Part model, mm, in its own coordinate system. Give positions to 0.01 mm unless a question says otherwise; leave off trailing zeros. Order: outer loops, then holes, each group sorted by start corner. A loop starts at its lowest first (then second) coordinate and runs counter-clockwise, first axis right, second up. Notation, with made-up numbers: M 65.5,13.5 L 78.5,13.5 A27 cw 78.5,35.5 Z; hole C 64,27.25 d5. An arc over 180 degrees is marked long. Answer as a JSON object with one key per item and string values.
from build123d import *

# Parameters (mm, degrees)
SKETCH2_R           = 1.65
SKETCH2_R_2         = 11
SKETCH2_R_3         = 2.25
BOSS_EXTRUDE1_DEPTH = 3.8


with BuildPart() as part:
    # Sketch2 → Boss-Extrude1 (new body)
    with BuildSketch(Plane.XY):
        with BuildLine():
            Line((-160, 155), (-87, 155))
            ThreePointArc((-87, 155), (-85.585786438, 154.414213562), (-85, 153))
            Line((-85, 153), (-85, 74.308795954))
            ThreePointArc((-85, 74.308795954), (-84.414213562, 72.894582392), (-83, 72.308795954))
            Line((-83, 72.308795954), (83, 72.308795954))
            ThreePointArc((83, 72.308795954), (84.414213562, 72.894582392), (85, 74.308795954))
            Line((85, 74.308795954), (85, 153))
            ThreePointArc((85, 153), (85.585786438, 154.414213562), (87, 155))
            Line((87, 155), (160, 155))
            Line((160, 155), (160, 55))
            Line((160, 55), (155, 55))
            Line((155, 55), (155, -5))
            Line((155, -5), (160, -5))
            Line((160, -5), (160, -105))
            Line((160, -105), (87, -105))
            ThreePointArc((87, -105), (85.585786438, -104.414213562), (85, -103))
            Line((85, -103), (85, -22))
            ThreePointArc((85, -22), (84.414213562, -20.585786438), (83, -20))
            Line((83, -20), (-83, -20))
            ThreePointArc((-83, -20), (-84.414213562, -20.585786438), (-85, -22))
            Line((-85, -22), (-85, -103))
            ThreePointArc((-85, -103), (-85.585786438, -104.414213562), (-87, -105))
            Line((-87, -105), (-160, -105))
            Line((-160, -105), (-160, -5))
            Line((-160, -5), (-155, -5))
            Line((-155, -5), (-155, 55))
            Line((-155, 55), (-160, 55))
            Line((-160, 55), (-160, 155))
        make_face()
        with Locations(Location((-108.992804496, 124.770936608, 0), (0, 0, 180))):
            Circle(SKETCH2_R, mode=Mode.SUBTRACT)
        with Locations(Location((-108.992804496, 96.101330956, 0), (0, 0, 180))):
            Circle(SKETCH2_R, mode=Mode.SUBTRACT)
        with Locations(Location((108.992804496, 124.770936608, 0), (0, 0, 180))):
            Circle(SKETCH2_R, mode=Mode.SUBTRACT)
        with Locations(Location((108.992804496, 96.101330956, 0), (0, 0, 180))):
            Circle(SKETCH2_R, mode=Mode.SUBTRACT)
        with Locations(Location((108.992804496, 110.436133782, 0), (0, 0, 180))):
            Circle(SKETCH2_R_2, mode=Mode.SUBTRACT)
        with Locations(Location((-108.992804496, 110.436133782, 0), (0, 0, 180))):
            Circle(SKETCH2_R_2, mode=Mode.SUBTRACT)
        with Locations(Location((143.59774802, -0.5, 0), (0, 0, 180))):
            Circle(SKETCH2_R, mode=Mode.SUBTRACT)
        with Locations(Location((143.59774802, 50.5, 0), (0, 0, 180))):
            Circle(SKETCH2_R, mode=Mode.SUBTRACT)
        with Locations(Location((-143.59774802, -0.5, 0), (0, 0, 180))):
            Circle(SKETCH2_R, mode=Mode.SUBTRACT)
        with Locations(Location((-143.59774802, 50.5, 0), (0, 0, 180))):
            Circle(SKETCH2_R, mode=Mode.SUBTRACT)
        with Locations(Location((-47, 10.055, 0), (0, 0, 180))):
            Circle(SKETCH2_R_3, mode=Mode.SUBTRACT)
        with Locations(Location((-47, 39.945, 0), (0, 0, 180))):
            Circle(SKETCH2_R_3, mode=Mode.SUBTRACT)
        with Locations(Location((-71.06, 39.945, 0), (0, 0, 180))):
            Circle(SKETCH2_R_3, mode=Mode.SUBTRACT)
        with Locations(Location((-71.06, 10.055, 0), (0, 0, 180))):
            Circle(SKETCH2_R_3, mode=Mode.SUBTRACT)
        with Locations(Location((71.06, 10.055, 0), (0, 0, 180))):
            Circle(SKETCH2_R_3, mode=Mode.SUBTRACT)
        with Locations(Location((47, 10.055, 0), (0, 0, 180))):
            Circle(SKETCH2_R_3, mode=Mode.SUBTRACT)
        with Locations(Location((47, 39.945, 0), (0, 0, 180))):
            Circle(SKETCH2_R_3, mode=Mode.SUBTRACT)
        with Locations(Location((71.06, 39.945, 0), (0, 0, 180))):
            Circle(SKETCH2_R_3, mode=Mode.SUBTRACT)
        with Locations(Location((108.992804496, -74.770936608, 0), (0, 0, 180))):
            Circle(SKETCH2_R, mode=Mode.SUBTRACT)
        with Locations(Location((108.992804496, -46.101330956, 0), (0, 0, 180))):
            Circle(SKETCH2_R, mode=Mode.SUBTRACT)
        with Locations(Location((108.992804496, -60.436133782, 0), (0, 0, 180))):
            Circle(SKETCH2_R_2, mode=Mode.SUBTRACT)
        with Locations(Location((-108.992804496, -60.436133782, 0), (0, 0, 180))):
            Circle(SKETCH2_R_2, mode=Mode.SUBTRACT)
        with Locations(Location((-108.992804496, -46.101330956, 0), (0, 0, 180))):
            Circle(SKETCH2_R, mode=Mode.SUBTRACT)
        with Locations(Location((-108.992804496, -74.770936608, 0), (0, 0, 180))):
            Circle(SKETCH2_R, mode=Mode.SUBTRACT)
        with Locations(Location((38.179918963, -11.563765186, 0), (0, 0, 180))):
            Circle(SKETCH2_R_3, mode=Mode.SUBTRACT)
        with Locations(Location((-38.179918963, -11.563765186, 0), (0, 0, 180))):
            Circle(SKETCH2_R_3, mode=Mode.SUBTRACT)
        with BuildLine():
            Line((-84, 62.171403079), (-129.59774802, 62.171403079))
            ThreePointArc((-129.59774802, 62.171403079), (-132.426175145, 60.999830204), (-133.59774802, 58.171403079))
            Line((-133.59774802, 58.171403079), (-133.59774802, -8.171403079))
            ThreePointArc((-133.59774802, -8.171403079), (-132.426175145, -10.999830204), (-129.59774802, -12.171403079))
            Line((-129.59774802, -12.171403079), (-84, -12.171403079))
            ThreePointArc((-84, -12.171403079), (-81.171572875, -10.999830204), (-80, -8.171403079))
            Line((-80, -8.171403079), (-80, 58.171403079))
            ThreePointArc((-80, 58.171403079), (-81.171572875, 60.999830204), (-84, 62.171403079))
        make_face(mode=Mode.SUBTRACT)
        with BuildLine():
            Line((84, 62.171403079), (129.59774802, 62.171403079))
            ThreePointArc((129.59774802, 62.171403079), (132.426175145, 60.999830204), (133.59774802, 58.171403079))
            Line((133.59774802, 58.171403079), (133.59774802, -8.171403079))
            ThreePointArc((133.59774802, -8.171403079), (132.426175145, -10.999830204), (129.59774802, -12.171403079))
            Line((129.59774802, -12.171403079), (84, -12.171403079))
            ThreePointArc((84, -12.171403079), (81.171572875, -10.999830204), (80, -8.171403079))
            Line((80, -8.171403079), (80, 58.171403079))
            ThreePointArc((80, 58.171403079), (81.171572875, 60.999830204), (84, 62.171403079))
        make_face(mode=Mode.SUBTRACT)
    extrude(amount=BOSS_EXTRUDE1_DEPTH)


solid = part.part
1. Cut at C-C on y = 19.5. Give the cut face in (x, z).
Worked answers:
{"outline": "M -155,0 L -133.6,0 L -133.6,3.8 L -155,3.8 Z; M -80,0 L 80,0 L 80,3.8 L -80,3.8 Z; M 133.6,0 L 155,0 L 155,3.8 L 133.6,3.8 Z"}
2. Pin check, flat tips, straight feed: P1, Ø1, axis at x = -26, z = 1, coming from the -Y side; P2, Ø3.5, axis at x = 47, y = 10.055, coming from the -Z side; P3, Ø1.5, axis at x = -31.5, z = 2, coming from the +Y side. Stop position of each tip, or through.
Worked answers:
{"P1": "stops at y = -20", "P2": "passes through", "P3": "stops at y = 72.31"}
3. Cut at A-A on x = -93. Give the cut face in (y, z).
Worked answers:
{"outline": "M -105,0 L -12.17,0 L -12.17,3.8 L -105,3.8 Z; M 62.17,0 L 155,0 L 155,3.8 L 62.17,3.8 Z"}
4. Cut at B-B on y = 78. Give the cut face in (x, z), plus the area to 3 significant figures.
Worked answers:
{"outline": "M -160,0 L -85,0 L -85,3.8 L -160,3.8 Z; M 85,0 L 160,0 L 160,3.8 L 85,3.8 Z", "area": "570 mm^2"}
5. Cut at D-D on y = 114.5. Give the cut face in (x, z).
Worked answers:
{"outline": "M -160,0 L -119.21,0 L -119.21,3.8 L -160,3.8 Z; M -98.77,0 L -85,0 L -85,3.8 L -98.77,3.8 Z; M 85,0 L 98.77,0 L 98.77,3.8 L 85,3.8 Z; M 119.21,0 L 160,0 L 160,3.8 L 119.21,3.8 Z"}
6. Two-plate mould, pull along X, no slides. Class faces 1 (the cylindrical face through (117.1, 103, 1.9)), 2 (the flat face through (2, 27, 3.8)): +X half, -X half, draft (parallel to the pull), parting line (faces both ways), or undercut.
Worked answers:
{"face 1": "undercut", "face 2": "draft"}
7. Probe line 1 along X through (y, z) = (23.5, 3.1); line 2 along Y through (x, z) = (-46.5, 3.55); line 3 along X through (y, z) = (109.5, 2.15). List the from-to ranges inside material, lowest first.
Worked answers:
{"line 1": "x = -155 to -133.6, -80 to 80, 133.6 to 155", "line 2": "y = -20 to 7.86, 12.25 to 37.75, 42.14 to 72.31", "line 3": "x = -160 to -119.95, -98.03 to -85, 85 to 98.03, 119.95 to 160"}
